The model under review builds one solid part; all positions refer to its coordinate system, in mm. A direction names the side the tool comes from. Round coordinates to 2 decimals unless told otherwise and drop trailing zeros. Loops run counter-clockwise (first coordinate to the right, second up) from the corner with the lowest first, then second, coordinate; pieces in that order, holes last. Notation, with made-up numbers: M 44,64.25 L 95,64.25 A12 ccw 95,81.25 Z; hole C -1,-18.75 d1. An arc over 180 degrees is marked long. Answer as a JSON object with one key per item and string values. Group by question number.
Item 1: The part is to be moulded in two halves that separate along Y. For faces 4 (the face through (-31.75, 53, 52)), 5 (the face through (43, 24.218, 9)), 6 (the face through (-1, 6.032, 63)), say which applies: +Y half, -Y half, draft (parallel to the pull), parting line (faces both ways), or undercut.
Item 2: Consider section C-C (y = 98). Give the boundary of the cut face in (x, z), and give its area (3 significant figures).
Item 3: Tool access review of faces 1 (the face through (51, 119.894, -3)), 2 (the face through (-29.95, 84.72, -27.47)), 3 (the face through (43, 12.686, 9)): name each direction out of +Z, -Z, +X, -X, +Y, -Y from which nothing blocks a thin tool from reaching the whole face with its end or side.
Item 4: Consider section D-D (y = 130.5). Give the boundary of the cut face in (x, z), and give its area (3 significant figures).
Item 5: To check wall thickness, follow line 1 (Z direction, x = 0, y = 68.5); line 2 (X direction, y = 94, z = 0); line 3 (Z direction, x = -19.5, y = 31.5). State the ranges of each line that lie inside material, in increasing order.
Item 6: Insertion check: P1, Ø5, axis at x = 33.5, z = 46.5, coming from the +Y side; P2, Ø4, axis at x = -5.5, z = 23.5, coming from the -Y side; P3, Ø5, axis at x = 32, y = 90.5, coming from the -Z side; P4, Ø8, axis at x = 26, y = 18.5, coming from the -Z side. Each pin has a flat end and moves straight along its axis. Give the tip position at first contact, or say it passes through.
Item 7: Consider section A-A (y = 58). Give the boundary of the cut face in (x, z).
Item 8: Consider section B-B (x = 58). Give the boundary of the cut face in (y, z).
Autodesk Inventor part; units mm, degrees
ref_plane "Work Plane2" through (46.5, 0, 0) normal (1, 0, 0) x (0, 1, 0)
ref_plane "Work Plane4" through (0, 0, 46.5) normal (0, 0, 1) x (1, 0, 0)
ref_plane "Work Plane5" through (46.5, 0, 0) normal (1, 0, 0) x (0, 1, 0)
sketch "Sketch1" plane through (0, 0, 0) normal (0, 1, 0) x (-1, 0, 0)
  circle A0 centre (0, 0) radius 46.5
  dimension "d0" = 93
extrude "Extrusion1" add sketch "Sketch1" along normal blind 90
sketch "Sketch2" plane through (0, 90, 0) normal (0, 1, 0) x (1, 0, 0)
  circle A0 centre (0, 0) radius 50.8
  dimension "d3" = 101.6
extrude "Extrusion2" add sketch "Sketch2" along normal blind 146.05
sketch "Sketch4" plane through (0, 90, 0) normal (0, -1, 0) x (1, 0, 0)
  point P0 (0, 0)
sketch "Sketch5" plane through (0, 90, 0) normal (0, -1, 0) x (1, 0, 0)
  point P0 (0, 0)
sketch "Sketch6" plane through (0, 90, 0) normal (0, -1, 0) x (1, 0, 0)
  point P0 (0, 0)
fillet "Fillet1" radius 2 2 edges at (-50.8, 90, 0) (46.5, 90, 0)
ref_plane "Work Plane2" through (46.5, 0, 0) normal (1, 0, 0) x (0, 1, 0)
sketch "Sketch7" plane through (46.5, 0, 0) normal (1, 0, 0) x (0, 1, 0)
  line L0 (24.2179, 0) -> (12.6856, 0)
  line L1 (12.6856, 0) -> (12.6856, 18.4517)
  line L2 (12.6856, 18.4517) -> (24.2179, 18.4517)
  line L3 (24.2179, 18.4517) -> (24.2179, 0)
  point P0 (0, 0)
extrude "Extrusion4" cut sketch "Sketch7" against normal blind 17.4625
sketch "Sketch12" plane through (0, 90, 0) normal (0, -1, 0) x (1, 0, 0)
  point P0 (0, 0)
sketch "Sketch13" plane through (0, 90, 0) normal (0, -1, 0) x (1, 0, 0)
  point P0 (0, 0)
sketch "Sketch14" plane through (0, 90, 0) normal (0, -1, 0) x (1, 0, 0)
  line L0 (65.7696, 29.9336) -> (57.3376, 29.9336)
  line L1 (57.3376, 29.9336) -> (57.3376, 7.1672)
  line L2 (57.3376, 7.1672) -> (65.7696, 7.1672)
  line L3 (65.7696, 7.1672) -> (65.7696, 29.9336)
  point P0 (0, 0)
extrude "Extrusion8" cut sketch "Sketch14" against normal blind 141.605
ref_plane "Work Plane4" through (0, 0, 46.5) normal (0, 0, 1) x (1, 0, 0)
sketch "Sketch24" plane through (0, 0, 46.5) normal (0, 0, 1) x (1, 0, 0)
  point P0 (0, 0)
sketch "Sketch25" plane through (0, 0, 46.5) normal (0, 0, 1) x (1, 0, 0)
  line L0 (0, 0) -> (-31.75, 0)
  line L1 (-31.75, 0) -> (-31.75, 104.14)
  line L2 (-31.75, 104.14) -> (0, 104.14)
  line L3 (0, 104.14) -> (0, 0)
  line L4 (0, 0) -> (31.75, 0)
  line L5 (31.75, 0) -> (31.75, 104.14)
  line L6 (31.75, 104.14) -> (0, 104.14)
  line L7 (0, 104.14) -> (0, 0)
  dimension "d59" = 31.75
  dimension "d60" = 104.14
  dimension "d61" = 31.75
  dimension "d62" = 104.14
extrude "Extrusion13" add sketch "Sketch25" along normal blind 33.02
sketch "Sketch26" plane through (0, 0, 79.52) normal (0, 0, 1) x (1, 0, 0)
  line L0 (-31.75, 104.14) -> (-31.75, 0)
  line L1 (0, 0) -> (31.75, 0)
  line L2 (-31.75, 104.14) -> (31.75, 104.14)
  line L3 (31.75, 104.14) -> (31.75, 0)
  line L4 (31.75, 0) -> (-31.75, 0)
  line L5 (-31.75, 0) -> (-31.75, 104.14)
extrude "Extrusion14" add sketch "Sketch26" against normal blind 44.7675
sketch "Sketch27" plane through (0, 104.14, 0) normal (0, 1, 0) x (1, 0, 0)
  point P0 (0, 0)
sketch "Sketch28" plane through (0, 104.14, 0) normal (0, 1, 0) x (1, 0, 0)
  point P0 (0, 0)
sketch "Sketch29" plane through (0, 104.14, 0) normal (0, 1, 0) x (1, 0, 0)
  line L0 (-28.6575, -50.7647) -> (27.2225, -50.7647)
  line L1 (27.2225, -50.7647) -> (27.2225, -76.1647)
  line L2 (27.2225, -76.1647) -> (-28.6575, -76.1647)
  line L3 (-28.6575, -76.1647) -> (-28.6575, -50.7647)
  point P0 (0, 0)
  dimension "d67" = 55.88
  dimension "d68" = 25.4
extrude "Extrusion15" cut sketch "Sketch29" against normal blind 98.1075
sketch "Sketch30" plane through (-31.75, 0, 79.52) normal (-1, 0, 0) x (0, 0, 1)
  line L0 (-0.5043, 102.352) -> (0, 76.957)
  line L1 (0, 0) -> (0, 104.14)
  line L2 (-24.2726, 76.475) -> (-9.0326, 76.475)
  line L3 (-9.0326, 76.475) -> (-9.0326, 38.375)
  line L4 (-9.0326, 38.375) -> (-24.2726, 38.375)
  line L5 (-24.2726, 38.375) -> (-24.2726, 76.475)
  point P0 (-79.52, 0)
  dimension "d71" = 25.4
  dimension "d72" = 15.24
  dimension "d73" = 38.1
extrude "Extrusion16" cut sketch "Sketch30" against normal blind 46.355
ref_plane "Work Plane5" through (46.5, 0, 0) normal (1, 0, 0) x (0, 1, 0)
sketch "Sketch31" plane through (46.5, 0, 0) normal (1, 0, 0) x (0, 1, 0)
  line L0 (11.9436, 0) -> (43.6936, 0)
  line L1 (43.6936, 0) -> (119.8936, 0)
  line L2 (119.8936, 0) -> (119.8936, 38.1)
  line L3 (119.8936, 38.1) -> (43.6936, 38.1)
  line L4 (43.6936, 38.1) -> (43.6936, 0)
  line L5 (43.6936, 0) -> (119.8936, 0)
  line L6 (119.8936, 0) -> (119.8936, -38.1)
  line L7 (119.8936, -38.1) -> (43.6936, -38.1)
  line L8 (43.6936, -38.1) -> (43.6936, 0)
  point P0 (0, 0)
  dimension "d76" = 31.75
  dimension "d77" = 76.2
  dimension "d78" = 38.1
  dimension "d79" = 76.2
  dimension "d80" = 38.1
extrude "Extrusion17" add sketch "Sketch31" along normal blind 25.4
sketch "Sketch32" plane through (71.9, 0, 0) normal (1, 0, 0) x (0, 0, -1)
  point P0 (0, 0)
sketch "Sketch33" plane through (71.9, 0, 0) normal (1, 0, 0) x (0, 0, -1)
  line L0 (-20.4546, 119.8936) -> (-38.1, 119.8936)
  line L1 (0, 43.6936) -> (38.1, 43.6936)
  line L2 (-38.1, 119.8936) -> (38.1, 119.8936)
  line L3 (38.1, 119.8936) -> (38.1, 43.6936)
  line L4 (38.1, 43.6936) -> (-38.1, 43.6936)
  line L5 (-38.1, 43.6936) -> (-38.1, 119.8936)
  point P0 (0, 0)
extrude "Extrusion18" add sketch "Sketch33" against normal blind 47.625
sketch "Sketch3" plane through (0, 236.05, 0) normal (0, 1, 0) x (1, 0, 0)
  circle A0 centre (0, 0) radius 40.64
  dimension "d6" = 81.28
extrude "Extrusion3" cut sketch "Sketch3" against normal blind 228.6
sketch "Sketch34" plane through (33.601, 119.8936, 38.1) normal (0, 1, 0) x (1, 0, 0)
  line L0 (34.9589, 72.1697) -> (18.4489, 72.1697)
  line L1 (18.4489, 72.1697) -> (18.4489, 3.5897)
  line L2 (18.4489, 3.5897) -> (34.9589, 3.5897)
  line L3 (34.9589, 3.5897) -> (34.9589, 72.1697)
  point P0 (-33.601, 38.1)
  dimension "d85" = 16.51
  dimension "d86" = 68.58
extrude "Extrusion19" cut sketch "Sketch34" against normal blind 71.4375
sketch "Sketch35" plane through (26.6578, 43.6936, -38.1) normal (0, -1, 0) x (1, 0, 0)
  point P0 (-26.6578, 38.1)
sketch "Sketch36" plane through (26.6578, 43.6936, -38.1) normal (0, -1, 0) x (1, 0, 0)
  line L0 (39.3784, 66.2811) -> (27.1807, 66.2811)
  line L1 (27.1807, 66.2811) -> (27.1807, 40.6237)
  line L2 (27.1807, 40.6237) -> (39.3784, 40.6237)
  line L3 (39.3784, 40.6237) -> (39.3784, 66.2811)
  point P0 (-26.6578, 38.1)
extrude "Extrusion20" cut sketch "Sketch36" against normal blind 71.4375
sketch "Sketch37" plane through (0, 236.05, 0) normal (0, 1, 0) x (1, 0, 0)
  circle A0 centre (0, 0) radius 58.234
extrude "Extrusion21" cut sketch "Sketch37" against normal blind 76.2
properties part number "_3DPrint"
Geometry results:
{
 "1": {"face 4": "draft", "face 5": "undercut", "face 6": "+Y half"},
 "2": {"outline": "M -31.75,39.66 A50.8 ccw long 33.6,-38.1 L 71.9,-38.1 L 71.9,38.1 L 33.6,38.1 A50.8 ccw 31.75,39.66 L 31.75,79.52 L -31.75,79.52 Z; hole C 0,0 d81.28; hole M -28.66,50.76 L 27.22,50.76 L 27.22,76.16 L -28.66,76.16 Z; hole M 52.05,-34.07 L 68.56,-34.07 L 68.56,34.51 L 52.05,34.51 Z", "area": "4,430 mm^2"},
 "3": {"face 1": "+X, +Y", "face 2": "+Y", "face 3": "+X"},
 "4": {"outline": "C 0,0 d101.6; hole C 0,0 d81.28", "area": "2,920 mm^2"},
 "5": {"line 1": "z = -46.5 to -40.64, 40.64 to 50.76, 76.16 to 79.52", "line 2": "x = -50.8 to -40.64, 40.64 to 52.05, 68.56 to 71.9", "line 3": "z = -42.21 to -35.66, 35.66 to 50.76, 76.16 to 79.52"},
 "6": {"P1": "stops at y = 104.14", "P2": "stops at y = 0", "P3": "stops at z = -41.13", "P4": "stops at z = -40.97"},
 "7": {"outline": "M -31.75,34.75 L -30.9,34.75 A46.5 ccw 26.66,-38.1 L 71.9,-38.1 L 71.9,38.1 L 31.75,38.1 L 31.75,79.52 L -31.75,79.52 L -31.75,70.49 L -28.66,70.49 L -28.66,76.16 L 27.22,76.16 L 27.22,50.76 L -28.66,50.76 L -28.66,55.25 L -31.75,55.25 Z; hole C 0,0 d81.28; hole M 52.05,-34.07 L 68.56,-34.07 L 68.56,34.51 L 52.05,34.51 Z"},
 "8": {"outline": "M 43.69,-38.1 L 119.89,-38.1 L 119.89,-34.07 L 48.46,-34.07 L 48.46,2.52 L 43.69,2.52 Z; M 43.69,28.18 L 48.46,28.18 L 48.46,34.51 L 119.89,34.51 L 119.89,38.1 L 43.69,38.1 Z"}
}
